from build123d import *

# Parameters (mm, degrees)
SKETCH_1_R          = 5
SKETCH_1_R_2        = 2.5
EXTRUDE_1_DEPTH     = 4.8
SKETCH_3_R          = 1.825
CUT_EXTRUDE_1_DEPTH = 2


with BuildPart() as part:
    # 스케치1 → 보스-돌출1 (new body)
    # profile 1 of 2: a face of its own
    with BuildSketch(Plane.XY):
        with BuildLine():
            ThreePointArc((5, 0), (0, -5), (-5, 0))
            Line((-5, 0), (-5, -2.326474397))
            Line((-5, -2.326474397), (0.754164722, -7.377840375))
            Line((0.754164722, -7.377840375), (0.754164722, -29.519890116))
            Line((0.754164722, -29.519890116), (2.889052882, -29.519890116))
            Line((2.889052882, -29.519890116), (4.518521564, -23.177422563))
            Line((4.518521564, -23.177422563), (7.08991094, -19.990348408))
            Line((7.08991094, -19.990348408), (7.08991094, -16.35629501))
            Line((7.08991094, -16.35629501), (6.40208237, -15.801342415))
            Line((6.40208237, -15.801342415), (6.40208237, -3.376138068))
            ThreePointArc((6.40208237, -3.376138068), (6.694975589, -2.669031287), (7.40208237, -2.376138068))
            Line((7.40208237, -2.376138068), (18.043960793, -2.376138068))
            Line((18.043960793, -2.376138068), (19.056002599, 4.757997197))
            Line((19.056002599, 4.757997197), (1.536705134, 4.757997197))
            ThreePointArc((1.536705134, 4.757997197), (4.04249463, 2.942488261), (5, 0))
        make_face()
    # profile 2 of 2: a face of its own
    with BuildSketch(Plane.XY):
        Circle(SKETCH_1_R)
        Circle(SKETCH_1_R_2, mode=Mode.SUBTRACT)
    extrude(amount=EXTRUDE_1_DEPTH)

    # 스케치3 → 컷-돌출1 (cut)
    with BuildSketch(Plane.ZY.offset(-0.754164722)):
        with Locations((2.4, -27.019890116)):
            Circle(SKETCH_3_R)
    extrude(amount=-CUT_EXTRUDE_1_DEPTH, mode=Mode.SUBTRACT)


solid = part.part
Can you work these out from the model? Positions are in its coordinate system, mm. A direction names the side the tool comes from. Coordinates: 2 decimals unless noted, no trailing zeros. Loops run counter-clockwise (first coordinate to the right, second up) from the corner with the lowest first, then second, coordinate; pieces in that order, holes last. Notation, with made-up numbers: (-36, 64.25) - (-27, 64.25) arc R15 ccw to (-27, 71.25) - close; hole circle Ø7 at (22, 8.5). An arc over 180 degrees is marked (long way). Answer as a JSON object with one key per item and string values. Group by question number.
Item 1: For pin 1 (1.5 mm diameter, centred on y = -21, z = 3, fed in from -X); pin 2 (1.4 mm diameter, centred on x = 13.5, z = 2.5, fed in from +Y); pin 3 (1.4 mm diameter, centred on x = 12, z = 3.5, fed in from -Y), each with a flat end and sliding along its axis, tell me the tip position at first contact or that it passes through.
Item 2: If I drill on L1, parallel to Y at x = 2.1, z = 2.4; L2, parallel to Y at x = 1.55, z = 2.4; L3, parallel to Y at x = 7.5, z = 3.65, over which ranges is the centre line in solid material (lowest first)? Write a range as from..to.
Item 3: If we section it at B-B (x = 0): List the corners of the cut face in (y, z) for me, plus the area to 3 significant figures.
Item 4: If we section it at A-A (z = 2.4): List the corners of the cut face in (x, y) for me.
Item 5: On a 3-axis mill with a long thin cutter (end or side, diameter ignored), from which of +Z, -Z, +X, -X, +Y, -Y can I reach the whole of each face in a straight line? I mean faces 4 (the face through (10, 4.758, 2)), 5 (the face through (13, -2.376, 2)), 6 (the face through (6.402, -10, 2)), 7 (the face through (0.754, -18, 2)). Say none if no direction works.
Item 6: If we section it at D-D (x = 12.75): List the corners of the cut face in (y, z) for me, plus the area to 3 significant figures.
Item 7: If we mould it in two halves opening along Z, with no side actions, what happens to faces 1 (the face through (2.754, -27, 2)), 2 (the face through (4, -8, 0)), 3 (the face through (6.687, -2.677, 2.366))? For each: released by +Z, released by -Z, zero draft, split by the parting line, or undercut.
Item 8: If we section it at C-C (y = -14): List the corners of the cut face in (x, z) for me.
Returned:
{
 "1": {"pin 1": "stops at x = 0.75", "pin 2": "stops at y = 4.76", "pin 3": "stops at y = -2.38"},
 "2": {"L1": "y = -29.52..-28.84, -25.19..-1.36, 1.36..4.76", "L2": "y = -29.52..-28.84, -25.19..-1.96, 1.96..4.76", "L3": "y = -2.38..4.76"},
 "3": {"outline": "(-6.72, 0) - (-2.5, 0) - (-2.5, 4.8) - (-6.72, 4.8) - close; (2.5, 0) - (5, 0) - (5, 4.8) - (2.5, 4.8) - close", "area": "32.2 mm²"},
 "4": {"outline": "(-5, -2.33) - (0.75, -7.38) - (0.75, -25.19) - (2.75, -25.19) - (2.75, -28.84) - (0.75, -28.84) - (0.75, -29.52) - (2.89, -29.52) - (4.52, -23.18) - (7.09, -19.99) - (7.09, -16.36) - (6.4, -15.8) - (6.4, -3.38) arc R1 cw to (7.4, -2.38) - (18.04, -2.38) - (19.06, 4.76) - (1.54, 4.76) arc R5 ccw to (-5, 0) - close; hole circle Ø5 at (0, 0)"},
 "5": {"face 4": "+Z, -Z, +X, +Y", "face 5": "+Z, -Z, +X, -Y", "face 6": "+Z, -Z, +X", "face 7": "+Z, -Z, -X, -Y"},
 "6": {"outline": "(-2.38, 0) - (4.76, 0) - (4.76, 4.8) - (-2.38, 4.8) - close", "area": "34.2 mm²"},
 "7": {"face 1": "undercut", "face 2": "released by -Z", "face 3": "zero draft"},
 "8": {"outline": "(0.75, 0) - (6.4, 0) - (6.4, 4.8) - (0.75, 4.8) - close"}
}
